Geometry: see drawing. Coordinates: mm, zero at the bounding-box minimum. A direction names the side the tool comes from. Give positions to 0.01 mm unless a question says otherwise; leave off trailing zeros. Loops run counter-clockwise (first coordinate to the right, second up) from the corner with the lowest first, then second, coordinate; pieces in that order, holes last. Notation, with made-up numbers: (-0.5, 65) - (21.5, 65) arc R6 ccw to (21.5, 75) - close; hole circle Ø6 at (74.25, 10.25). An arc over 180 degrees is marked (long way). One line per question, with ' | ' between items. Start each with the question number.
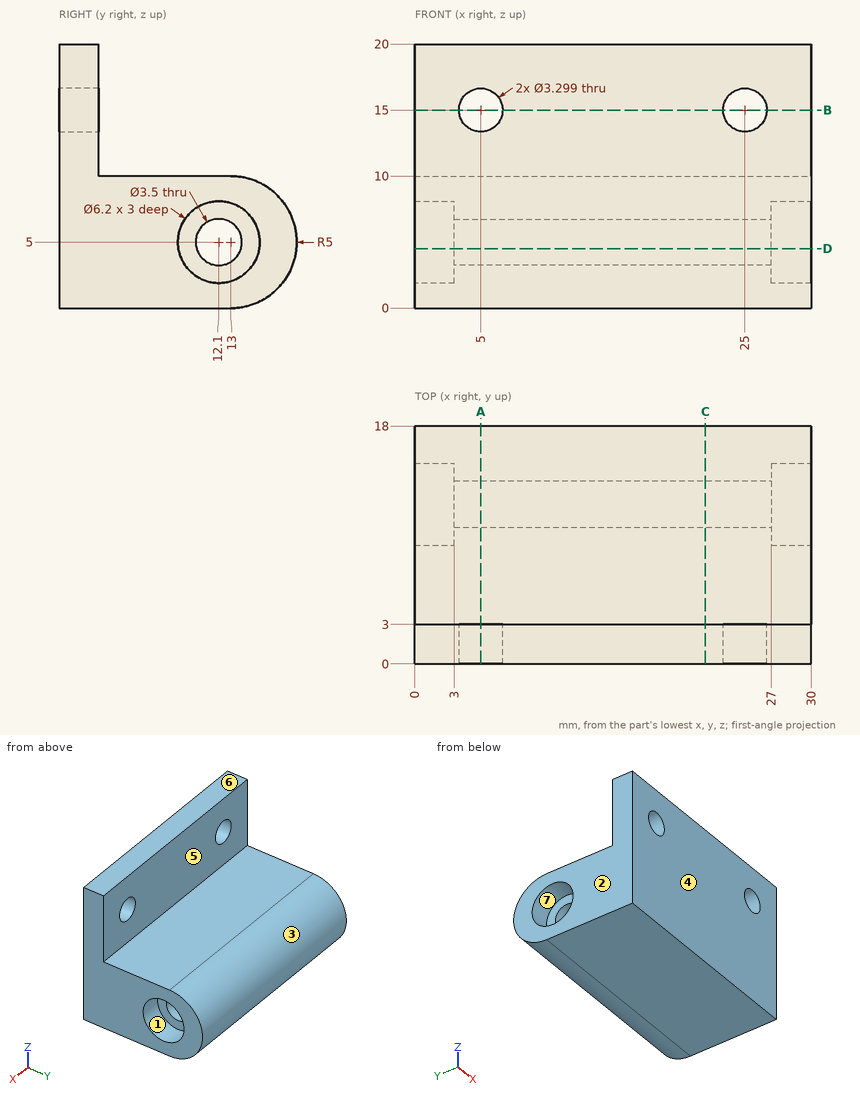
Q1. Section C-C, the plane x = 22. Output: boundary loops of the cut face in (y, z), plus the area to 3 significant figures.
Q2. Section B-B, the plane z = 15. Output: boundary loops of the cut face in (x, y), plus the area to 3 significant figures.
Q3. Section A-A, the plane x = 5. Output: boundary loops of the cut face in (y, z), plus the area to 3 significant figures.
Q4. Line query: L1, parallel to X at y = 1.5, z = 15; L2, parallel to Y at x = 2.75, z = 5; L3, parallel to Z at x = 2.3, y = 12.1. Output: solid intervals per line, ascending. Write a range as from..to.
Q5. First-contact query: pin 1 (2.5 mm diameter, centred on x = 5, z = 15, fed in from -Y); pin 2 (3 mm diameter, centred on x = 18, y = 9.5, fed in from +Z); pin 3 (4 mm diameter, centred on y = 12.1, z = 5, fed in from -X); pin 4 (8 mm diameter, centred on x = 16, z = 16.5, fed in from +Y). Flat tips, straight axial feed; report the tip coordinate or a pass-through.
Q6. Section D-D, the plane z = 4.5. Output: boundary loops of the cut face in (x, y) (1 decimal).
Q7. Draft query along Y for the marked faces 1, 2, 3 and 4. Return one class per face: +Y half, -Y half, draft (parallel to the pull), parting line (faces both ways), or undercut.
Q8. Access query for the marked faces 5, 6 and 7. Directions: +Z, -Z, +X, -X, +Y, -Y. A direction counts if a zero-diameter tool reaches every point of the face in a straight line with its end or side. Return the directions, or none.
Solved:
1) outline: (0, 0) - (13, 0) arc R5 ccw to (13, 10) - (3, 10) - (3, 20) - (0, 20) - close; hole circle Ø3.5 at (12.1, 5) | area: 190 mm²
2) outline: (0, 0) - (3.35, 0) - (3.35, 3) - (0, 3) - close; (6.65, 0) - (23.35, 0) - (23.35, 3) - (6.65, 3) - close; (26.65, 0) - (30, 0) - (30, 3) - (26.65, 3) - close | area: 70.2 mm²
3) outline: (0, 0) - (13, 0) arc R5 ccw to (13, 10) - (3, 10) - (3, 13.35) - (0, 13.35) - close; (0, 16.65) - (3, 16.65) - (3, 20) - (0, 20) - close; hole circle Ø3.5 at (12.1, 5) | area: 180 mm²
4) L1: x = 0..3.35, 6.65..23.35, 26.65..30 | L2: y = 0..9, 15.2..18 | L3: z = 0..1.9, 8.1..10
5) pin 1: passes through | pin 2: stops at z = 10 | pin 3: stops at x = 3 | pin 4: stops at y = 3
6) outline: (0, 0) - (30, 0) - (30, 9) - (27, 9) - (27, 10.4) - (3, 10.4) - (3, 9) - (0, 9) - close; (0, 15.2) - (3, 15.2) - (3, 13.8) - (27, 13.8) - (27, 15.2) - (30, 15.2) - (30, 18) - (0, 18) - close
7) face 1: undercut | face 2: draft | face 3: +Y half | face 4: -Y half
8) face 5: +Z, +X, -X, +Y | face 6: +Z, +X, -X, +Y, -Y | face 7: -X
